Autodesk Inventor part; units mm, degrees
ref_plane "Work Plane1" through (0, -20, 97) normal (0, 1, 0) x (-1, 0, 0)
ref_plane "YZ Plane" through (0, 0, 0) normal (1, 0, 0) x (0, 1, 0)
ref_plane "XY Plane" through (0, 0, 0) normal (0, 0, 1) x (1, 0, 0)
sketch "Sketch1" plane through (0, 0, 0) normal (1, 0, 0) x (0, 1, 0)
  line L0 (20, 97) -> (-20, 97) construction
  line L1 (-20, 97) -> (-20, -97) construction
  line L2 (-20, -97) -> (20, -97) construction
  line L3 (20, -97) -> (20, 97) construction
  line L4 (20, 97) -> (-20, -97) construction
  line L5 (-20, 97) -> (20, -97) construction
  line L6 (-20, 97) -> (19, 97)
  line L7 (-20, -97) -> (19, -97)
  arc A0 (20, 95.9982) -> (19, 97) centre (19, 96) ccw
  arc A1 (19, -97) -> (20, -95.9993) centre (19, -96) ccw
  line L8 (20, 95.9982) -> (20, -95.9993)
  point P0 (0, 0)
  dimension "d0" = 40
  dimension "d1" = 194
  dimension "d2" = 39
  dimension "d3" = 39
ref_plane "Work Plane1" through (0, -20, 97) normal (0, 1, 0) x (-1, 0, 0)
sketch "Sketch2" plane through (0, -20, 97) normal (0, 1, 0) x (-1, 0, 0)
  line L0 (0, 0) -> (40, 0)
  line L1 (40, 0) -> (40, -0.1)
  line L2 (40, -0.1) -> (0, -0.1)
  line L3 (0, -0.1) -> (0, 0)
  point P0 (0, -97)
  dimension "d4" = 40
  dimension "d5" = 0.1
sweep "Sweep1" add profiles "Sketch2" path "Sketch1"
sketch "Sketch3" plane through (-40, 20, 95.9982) normal (0, 1, 0) x (1, 0, 0)
  line L0 (0, -0.0002) -> (0, 191.9975) construction
  line L1 (40, 0) -> (40, -1.0018) construction
  line L2 (0, 191.9975) -> (40, 0) construction
  line L3 (40, -0.0002) -> (40, 191.9975) construction
  line L4 (40, 191.9975) -> (0, -0.0002) construction
  point P0 (40, 95.9982)
  point P1 (20, 95.9987)
hole "Hole1" at (-20, 20, -0.0004) direction (0, -1, 0) diameter 3 end through all
fillet "Fillet1" radius 2 4 edges at (0, -20, 96.95) (0, -19.9999, -96.95) (-40, -20, 96.95) (-40, -19.9999, -96.95)
sketch "Sketch4" plane through (-40, 19, 97) normal (0, 0, 1) x (1, 0, 0)
  line L0 (0, -37) -> (0, 0)
  line L1 (38, -39) -> (2, -39)
  point P0 (40, -19)
  point P1 (20, -29)
  dimension "d16" = 20
  dimension "d17" = 10
hole "Hole2" at (-20, -10, 97) direction (0, 0, -1) diameter 3 end through all
equation "\"d3\" = d2"
properties material "Iron, Malleable"
Read the model definition and answer for the solid it produces. Units are mm, in the model's axes. Give positions to 0.01 mm unless a question says otherwise; leave off trailing zeros. Write each loop counter-clockwise with the first axis right and the second up, starting at its lowest first coordinate (ties: lowest second). Pieces come first, ordered by that corner, then holes. Notation, with made-up numbers: M 51.5,-40 L 82.5,-40 A19 cw 82.5,-18 Z; hole C 85.25,53 d6. An arc over 180 degrees is marked long. One line per item, written item: value. Start each with the question number.
(1) Find section A-A (y = -16). Determine the outline of the cut face in (x, z).
(2) Find section B-B (x = -15). Determine the outline of the cut face in (y, z), plus the area to 3 significant figures.
(3) Find section C-C (z = 57.5). Determine the outline of the cut face in (x, y).
(4) Flat-ended cylindrical pins translate along their axes: pin 1 Ø2.5 at (x, y) = (-20, -10) entering from +Z; pin 2 Ø1.5 at (x, z) = (-22, 52.5) entering from -Y. Find the tip coordinate at first contact, or state that the pin passes through.
Results below:
1. outline: M -40,-97 L 0,-97 L 0,-96.9 L -40,-96.9 Z; M -40,96.9 L 0,96.9 L 0,97 L -40,97 Z
2. outline: M -20,-97 L 19,-97 A1 ccw 20,-96 L 20,96 A1 ccw 19,97 L -20,97 L -20,96.9 L 19,96.9 A0.9 cw 19.9,96 L 19.9,-96 A0.9 cw 19,-96.9 L -20,-96.9 Z
2. area: 27.3 mm^2
3. outline: M -40,19.9 L 0,19.9 L 0,20 L -40,20 Z
4. pin 1: passes through
4. pin 2: stops at y = 19.9
